Check sheet for the modelled part. Datum: model origin and axes. Units: mm. A direction names the side the tool comes from. Round coordinates to 2 decimals unless told otherwise and drop trailing zeros. Write each loop counter-clockwise with the first axis right and the second up, starting at its lowest first coordinate (ties: lowest second). Pieces come first, ordered by that corner, then holes. Notation, with made-up numbers: M 5,70.25 L 12,70.25 A33 cw 12,108.25 Z; hole C 62,-6 d7. An arc over 180 degrees is marked long. Put each result on its own line as item: value.
```python
from build123d import *

# Parameters (mm, degrees)
F0_W            = 95
F0_H            = 45
F1_DEPTH        = 1250
F2_W            = 95
F2_H            = 250
F3_DEPTH        = 45
F5_DEPTH        = 5
F5_COPIES_COUNT = 3
F5_COPIES_PITCH = 400
F8_DEPTH        = 5
F11_DEPTH       = 5
F13_DEPTH       = 45


# Not quite as in the source:
# - a pattern or mirror of a feature is missing from the dataset's text; its kind, count and spacing are read off the source's solid


with BuildPart() as f1:
    # F0 (on Front) → F1 (new body, symmetric)
    with BuildSketch(Plane.XZ):
        Rectangle(F0_W, F0_H)
    extrude(amount=F1_DEPTH, both=True)

    # F2 (on face) → F3 (cut, through all)
    with BuildSketch(Plane.XY.offset(22.5)):
        with Locations((0, 1125)):
            Rectangle(F2_W, F2_H)
        Polygon((47.5, -1250), (47.5, -1000), (-47.5, -905), (-47.5, -1250), align=None)
    extrude(amount=-F3_DEPTH, mode=Mode.SUBTRACT)

    # F4 (on Front) → F5 (cut, symmetric)
    with BuildSketch(Plane.XZ):
        Polygon((47.5, 22.5), (2.5, 22.5), (2.5, 7.5), (32.5, 7.5), (32.5, -22.5), (47.5, -22.5), align=None)
    f5 = extrude(amount=F5_DEPTH, both=True, mode=Mode.SUBTRACT)

    # F5_copies: F5 ×3
    with Locations(*[(0, i * F5_COPIES_PITCH, 0) for i in range(1, F5_COPIES_COUNT)]):
        add(f5, mode=Mode.SUBTRACT)

    # F7 (on offset) → F8 (cut, symmetric)
    with BuildSketch(Plane.XZ.offset(800)):
        Polygon((2.5, 22.5), (2.5, 7.5), (32.5, 7.5), (32.5, -22.5), (47.5, -22.5), (47.5, 22.5), align=None)
    extrude(amount=F8_DEPTH, both=True, mode=Mode.SUBTRACT)

    # F10 (on offset) → F11 (cut, symmetric)
    with BuildSketch(Plane.XZ.offset(400)):
        Polygon((2.5, 22.5), (2.5, 7.5), (32.5, 7.5), (32.5, -22.5), (47.5, -22.5), (47.5, 22.5), align=None)
    extrude(amount=F11_DEPTH, both=True, mode=Mode.SUBTRACT)

    # F12 (on face) → F13 (join, through all)
    with BuildSketch(Plane.XY.offset(22.5)):
        Polygon((0, -952.5), (-47.5, -905), (-47.5, -919.1421356237), (-7.0710678119, -959.5710678119), align=None)
    extrude(amount=-F13_DEPTH)


solid = f1.part
```
1. Depth check by flat-ended pin: pin 1 Ø4 at (x, z) = (7.5, -16.5) entering from -Y; pin 2 Ø3 at (y, z) = (-401, 17) entering from +X; pin 3 Ø5 at (x, y) = (21.5, 398.5) entering from +Z. Enter the tip coordinate at first touch or a pass-through.
Computed values:
pin 1: stops at y = -962
pin 2: stops at x = 2.5
pin 3: stops at z = 7.5
2. Scan lines: probe 1 along Y at (x, z) = (39.5, -20); probe 2 along Y at (x, z) = (6, 8); probe 3 along Y at (x, z) = (-43, 6.5). Record each from-to range of solid material in increasing order.
Computed values:
probe 1: y = -992 to -805, -795 to -405, -395 to -5, 5 to 395, 405 to 795, 805 to 1000
probe 2: y = -958.5 to -805, -795 to -405, -395 to -5, 5 to 395, 405 to 795, 805 to 1000
probe 3: y = -923.64 to 1000
3. Cross-section at B-B (x = -25). Enter the section's corners in (y, z).
Computed values:
outline: M -941.64,-22.5 L 1000,-22.5 L 1000,22.5 L -941.64,22.5 Z
4. Access from +Z, -Z, +X, -X, +Y, -Y to the whole of each face (thin tool, end or side, straight path). Record for faces 5 (the flat face through (47.5, -904, 0)), 6 (the flat face through (30, 405, 10)).
Computed values:
face 5: +Z, -Z, +X, +Y, -Y
face 6: +Z, +X
5. Cross-section at A-A (z = -13.5). Enter the section's corners in (x, y).
Computed values:
outline: M -47.5,-919.14 L -7.07,-959.57 L 0,-952.5 L 47.5,-1000 L 47.5,-805 L 32.5,-805 L 32.5,-795 L 47.5,-795 L 47.5,-405 L 32.5,-405 L 32.5,-395 L 47.5,-395 L 47.5,-5 L 32.5,-5 L 32.5,5 L 47.5,5 L 47.5,395 L 32.5,395 L 32.5,405 L 47.5,405 L 47.5,795 L 32.5,795 L 32.5,805 L 47.5,805 L 47.5,1000 L -47.5,1000 Z
6. Release check for a two-part mould opening along Y. For faces 1 (the flat face through (30, -5, 10)), 2 (the flat face through (47.5, -203, 0)), 3 (the flat face through (-1, 1000, 0)), 4 (the flat face through (24.1, -976.6, 0.3)) record: +Y half, -Y half, draft (parallel to the pull), parting line (faces both ways), or undercut.
Computed values:
face 1: undercut
face 2: draft
face 3: +Y half
face 4: -Y half
